For this review, use the dimensioned drawing (mm, ordinates from the lowest corner) and the shaded views. A direction names the side the tool comes from. Coordinates: 2 decimals unless noted, no trailing zeros. Loops run counter-clockwise (first coordinate to the right, second up) from the corner with the lowest first, then second, coordinate; pieces in that order, holes last. Notation, with made-up numbers: M 1.25,44 L 6.25,44 A31 ccw 6.25,82 Z; hole C -36,-24.75 d4. An arc over 180 degrees is marked long. Write item = value, one per line.
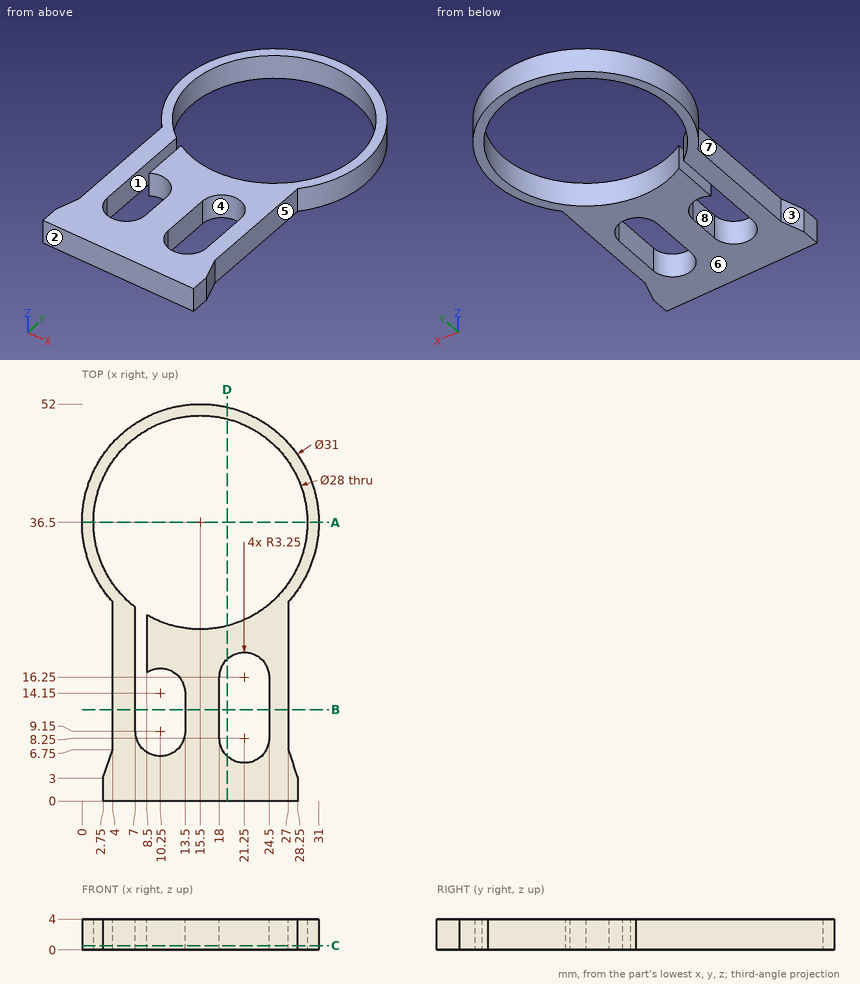
Q1. For pin 1 Ø1 at (y, z) = (28, 3) entering from -X; pin 2 Ø0.9 at (y, z) = (2, 1) entering from -X; pin 3 Ø2 at (y, z) = (24.5, 1) entering from -X, all flat-tipped, find the tip position at first contact; note any pin that passes through.
Solved:
pin_1 = 2.22
pin_2 = 2.75
pin_3 = 4
Q2. Add section B-B (y = 12). Write out the cut boundary in (x, z), and give its area (3 significant figures).
Solved:
outline = M 4,0 L 7,0 L 7,4 L 4,4 Z; M 13.5,0 L 18,0 L 18,4 L 13.5,4 Z; M 24.5,0 L 27,0 L 27,4 L 24.5,4 Z
area = 40.0 mm²
Q3. For line 1 along X through (y, z) = (11, 3.4); line 2 along X through (y, z) = (36.5, 1); line 3 along X through (y, z) = (24, 2.4), list the stretches that pass through material, from the lowest coordinate up.
Solved:
line_1 = 4 to 7, 13.5 to 18, 24.5 to 27
line_2 = 0 to 1.5, 29.5 to 31
line_3 = 4 to 7, 8.5 to 9.2, 21.8 to 27
Q4. Draft analysis for pull direction X (two halves, no side actions). For the marked faces 1, 2, 3 and 4, state which applies: +X half, -X half, draft (parallel to the pull), parting line (faces both ways), or undercut.
Solved:
face_1 = undercut
face_2 = draft
face_3 = -X half
face_4 = undercut
Q5. Add section D-D (x = 19). Write out the cut boundary in (y, z), and give its area (3 significant figures).
Solved:
outline = M 0,0 L 5.9,0 L 5.9,4 L 0,4 Z; M 18.6,0 L 22.94,0 L 22.94,4 L 18.6,4 Z; M 50.06,0 L 51.6,0 L 51.6,4 L 50.06,4 Z
area = 47.2 mm²
Q6. Machinability: for the marked faces 5, 6, 7 and 8, which of the approach directions +Z, -Z, +X, -X, +Y, -Y give a long, thin tool a straight path to every point of the face, cutting with its end or side? Answer none if there is none.
Solved:
face_5 = +Z, -Z, +X
face_6 = -Z, +X, -X, +Y, -Y
face_7 = +Z, -Z, -X
face_8 = +Z, -Z
Q7. Add section A-A (y = 36.5). Write out the cut boundary in (x, z).
Solved:
outline = M 0,0 L 1.5,0 L 1.5,4 L 0,4 Z; M 29.5,0 L 31,0 L 31,4 L 29.5,4 Z
Q8. Add section C-C (z = 0.55). Write out the cut boundary in (x, y), and give its area (3 significant figures).
Solved:
outline = M 2.75,0 L 28.25,0 L 28.25,3 L 27,6.75 L 27,26.11 A15.5 ccw long 4,26.11 L 4,6.75 L 2.75,3 Z; hole M 7,9.15 A3.25 ccw 13.5,9.15 L 13.5,14.15 A3.25 ccw 8.5,16.89 L 8.5,24.38 A14 ccw long 7,25.38 Z; hole M 18,8.25 A3.25 ccw 24.5,8.25 L 24.5,16.25 A3.25 ccw 18,16.25 Z
area = 506 mm²
